from build123d import *

# Parameters (mm, degrees)
F1_DEPTH = 30
F3_DEPTH = 8.001
F5_D     = 3


with BuildPart() as f1:
    # F0 (on Front) → F1 (new body)
    with BuildSketch(Plane.XZ):
        with BuildLine():
            Line((0, -3), (0, 0))
            Line((0, 0), (-26.6183650965, 0))
            Line((-26.6183650965, 0), (-26.7714593908, -0.8682408883))
            ThreePointArc((-26.7714593908, -0.8682408883), (-28.4815601075, -3.8302222156), (-31.6954981559, -5))
            Line((-31.6954981559, -5), (-32.5, -5))
            Line((-32.5, -5), (-32.5, -8))
            Line((-32.5, -8), (-24.9827011065, -8))
            Line((-24.9827011065, -8), (-24.8296068121, -7.1317591117))
            ThreePointArc((-24.8296068121, -7.1317591117), (-23.1195060955, -4.1697777844), (-19.905568047, -3))
            Line((-19.905568047, -3), (0, -3))
        make_face()
    extrude(amount=F1_DEPTH)

    # F2 (on face) → F3 (cut, through all)
    with BuildSketch(Plane.XY):
        with BuildLine():
            Line((0, -25), (0, -5))
            ThreePointArc((0, -5), (-10, -15), (0, -25))
        make_face()
        with BuildLine():
            ThreePointArc((0, -25), (7.0710678119, -22.0710678119), (10, -15))
            ThreePointArc((10, -15), (7.0710678119, -7.9289321881), (0, -5))
            Line((0, -5), (0, -25))
        make_face()
    extrude(amount=-F3_DEPTH, mode=Mode.SUBTRACT)

    # F5 (through all)
    with Locations(Plane(origin=(0, 0, -8), x_dir=(1, 0, 0), z_dir=(0, 0, -1))):
        with Locations((-29, 26.5), (-29, 3.5)):
            Hole(F5_D / 2)

    # F6: F1 across plane


with BuildPart() as f1_1:
    add(f1.part)
    add(f1.part.mirror(Plane.YZ))


solid = f1_1.part
Part model, mm, in its own coordinate system. A direction names the side the tool comes from. Coordinates: 2 decimals unless noted, no trailing zeros. Loops run counter-clockwise (first coordinate to the right, second up) from the corner with the lowest first, then second, coordinate; pieces in that order, holes last. Notation, with made-up numbers: (35.5, 61.5) -> (52.5, 61.5) arc R31 cw to (52.5, 94.5) -> close; hole circle Ø3 at (48.25, 48). An arc over 180 degrees is marked (long way). Use a Markdown table: item, result. Add a question column.
Item 1: Band-saw the part on B-B on y = -23. Write the cut outline in (x, z).
Item 2: Pull direction X, two halves, no side cores. Call faces 3 (the flat face through (-32.5, -15, -6)), 4 (the flat face through (29, -15, -8)), 5 (the cylindrical face through (-27.5, -26.57, -5.91)): +X half, -X half, draft (parallel to the pull), parting line (faces both ways), or undercut.
Item 3: Band-saw the part on D-D on z = -4.25. Write the cut outline in (x, y).
Item 4: Band-saw the part on A-A on x = 0. Write the cut outline in (y, z).
Item 5: Probe probe 1 along X at (y, z) = (-26.5, -5.9); probe 2 along X at (y, z) = (-3, -7); probe 3 along Z at (x, y) = (10, -4). List the from-to ranges inside material, lowest first.
Item 6: Flat gauge pins, fed straight in: P1, Ø3.5, axis at x = -29, y = -3.5, coming from the +Z side; P2, Ø4, axis at x = -18, y = -5.5, coming from the -Z side; P3, Ø1.5, axis at y = -26.5, z = -3.5, coming from the +X side. Where does each tip first touch, or does it go through?
Item 7: Band-saw the part on C-C on x = -29. Write the cut outline in (y, z).
Item 8: Which spindle directions (+Z, -Z, +X, -X, +Y, -Y) get a long thin tool onto all of the face, cutting with end or side? Do faces 1 (the cylindrical face through (-23.157, -14.79, -4.201)), 2 (the cylindrical face through (27.5, -3.57, -5.91)). Say none if no direction does.
Geometry says:
| question | item | result |
|---|---|---|
| 1 | outline | (-32.5, -8) -> (-24.98, -8) -> (-24.83, -7.13) arc R5 cw to (-19.91, -3) -> (-6, -3) -> (-6, 0) -> (-26.62, 0) -> (-26.77, -0.87) arc R5 cw to (-31.7, -5) -> (-32.5, -5) -> close; (6, -3) -> (19.91, -3) arc R5 cw to (24.83, -7.13) -> (24.98, -8) -> (32.5, -8) -> (32.5, -5) -> (31.7, -5) arc R5 cw to (26.77, -0.87) -> (26.62, 0) -> (6, 0) -> close |
| 2 | face 3 | -X half |
| 2 | face 4 | draft |
| 2 | face 5 | undercut |
| 3 | outline | (-29.06, -30) -> (-23.21, -30) -> (-23.21, 0) -> (-29.06, 0) -> (-29.06, -2) arc R1.5 cw (long way) to (-29.06, -5) -> (-29.06, -25) arc R1.5 cw (long way) to (-29.06, -28) -> close; (23.21, -30) -> (29.06, -30) -> (29.06, -28) arc R1.5 cw (long way) to (29.06, -25) -> (29.06, -5) arc R1.5 cw (long way) to (29.06, -2) -> (29.06, 0) -> (23.21, 0) -> close |
| 4 | outline | (-30, -3) -> (-25, -3) -> (-25, 0) -> (-30, 0) -> close; (-5, -3) -> (0, -3) -> (0, 0) -> (-5, 0) -> close |
| 5 | probe 1 | -32.5 to -30.5, -27.5 to -24.44, 24.44 to 27.5, 30.5 to 32.5 |
| 5 | probe 2 | -32.5 to -30.41, -27.59 to -24.8, 24.8 to 27.59, 30.41 to 32.5 |
| 5 | probe 3 | -3 to 0 |
| 6 | P1 | z = -2.29 |
| 6 | P2 | z = -3 |
| 6 | P3 | x = 27.7 |
| 7 | outline | (-30, -8) -> (-28, -8) -> (-28, -4.21) -> (-30, -4.21) -> close; (-25, -8) -> (-5, -8) -> (-5, -4.21) -> (-25, -4.21) -> close; (-2, -8) -> (0, -8) -> (0, -4.21) -> (-2, -4.21) -> close |
| 8 | face 1 | -Z, +Y, -Y |
| 8 | face 2 | +Z, -Z |
